Could you check a few things on this model? Use its own coordinates, in mm. Face numbers are marked on the shaded views. Give positions to 0.01 mm unless a question says otherwise; leave off trailing zeros. Order: outer loops, then holes, each group sorted by start corner. A loop starts at its lowest first (then second) coordinate and runs counter-clockwise, first axis right, second up.
(1) If I drill on probe 1 along X at (y, z) = (-11, 14.5); probe 2 along X at (y, z) = (-3, 1.25); probe 3 along Y at (x, z) = (-16, 14.75), over which ranges is the centre line in solid material (lowest first)?
(2) Imagine slicing it at A-A, the plane z = 7. Write out the boundary of the cut face in (x, y) (3 decimals), then the cut area to 3 significant figures.
(3) Imagine slicing it at B-B, the plane z = 1.75. Write out the boundary of the cut face in (x, y) (3 decimals).
(4) Will these pins go through, and if not, where does the flat tip stop? pin 1 (8 mm diameter, centred on x = 8, z = 23, fed in from -Y); pin 2 (3 mm diameter, centred on y = -15, z = 11, fed in from -X); pin 3 (6 mm diameter, centred on x = 1, z = 9.5, fed in from +Y).
(5) If we mould it in two halves opening along X, with no side actions, what happens to the marked faces 1, 2 and 3? For each: released by +X, released by -X, zero draft, split by the parting line, or undercut.
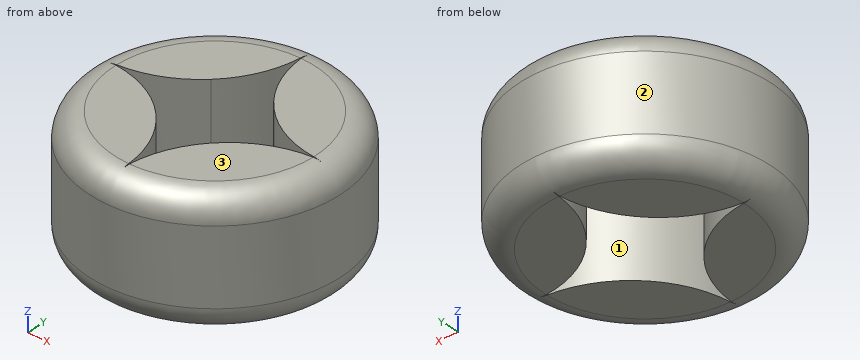
from build123d import *

# Parameters (mm, degrees)
F0_R     = 25.4
F1_DEPTH = 25.4


# Not quite as in the source:
# - a fillet or chamfer that OpenCascade refuses, or shapes differently, is made with other operations: its cross-section is extruded or revolved along the edge and cut away or added


with BuildPart() as f1:
    # F0 (on Top) → F1 (new body)
    with BuildSketch(Plane.XY):
        Circle(F0_R)
        with BuildLine():
            ThreePointArc((0, 22.225), (15.7154482119, 15.7154482119), (22.225, 0))
            ThreePointArc((22.225, 0), (15.7154482119, -15.7154482119), (0, -22.225))
            ThreePointArc((0, -22.225), (-15.7154482119, -15.7154482119), (-22.225, 0))
            ThreePointArc((-22.225, 0), (-15.7154482119, 15.7154482119), (0, 22.225))
        make_face(mode=Mode.SUBTRACT)
        with BuildLine():
            ThreePointArc((-6.5095517729, 6.5095518034), (-1.6917773858, 13.7198607256), (0, 22.225))
            ThreePointArc((0, 22.225), (-15.7154482119, 15.7154482119), (-22.225, 0))
            ThreePointArc((-22.225, 0), (-13.7198607057, 1.6917773941), (-6.5095517729, 6.5095518034))
        make_face()
        with BuildLine():
            ThreePointArc((6.509551813, 6.5095517633), (13.7198607319, 1.6917773832), (22.225, 0))
            ThreePointArc((22.225, 0), (15.7154482119, 15.7154482119), (0, 22.225))
            ThreePointArc((0, 22.225), (1.6917773967, 13.7198606994), (6.509551813, 6.5095517633))
        make_face()
        with BuildLine():
            ThreePointArc((-22.225, 0), (-15.7154482119, -15.7154482119), (0, -22.225))
            ThreePointArc((0, -22.225), (-1.6917773909, -13.7198607133), (-6.5095517917, -6.5095517845))
            ThreePointArc((-6.5095517917, -6.5095517845), (-13.719860718, -1.691777389), (-22.225, 0))
        make_face()
        with BuildLine():
            ThreePointArc((0, -22.225), (15.7154482119, -15.7154482119), (22.225, 0))
            ThreePointArc((22.225, 0), (13.7198607157, -1.6917773899), (6.5095517881, -6.5095517881))
            ThreePointArc((6.5095517881, -6.5095517881), (1.6917773899, -13.7198607157), (0, -22.225))
        make_face()
    extrude(amount=F1_DEPTH)

    # F2: fillet of radius 5.08 on 2 edges, made by hand

    # F2_s1 → F2_t2 (revolve, cut)
    with BuildSketch(Plane.XZ):
        with BuildLine():
            ThreePointArc((25.4, 20.32), (23.9121024484, 23.9121024484), (20.32, 25.4))
            Line((20.32, 25.4), (25.4, 25.4))
            Line((25.4, 25.4), (25.4, 20.32))
        make_face()
    revolve(axis=Axis((0, 0, 25.4), (0, 0, 1)), mode=Mode.SUBTRACT)

    # F2_s3 → F2_t4 (revolve, cut)
    with BuildSketch(Plane.XZ):
        with BuildLine():
            ThreePointArc((25.4, 5.08), (23.9121024484, 1.4878975516), (20.32, 0))
            Line((20.32, 0), (25.4, 0))
            Line((25.4, 0), (25.4, 5.08))
        make_face()
    revolve(axis=Axis((0, 0, 0), (0, 0, 1)), mode=Mode.SUBTRACT)


solid = f1.part
Answer block:
1. probe 1: x = -22.89 to -3.04, 3.04 to 22.89
1. probe 2: x = -23.47 to -11.07, 11.07 to 23.47
1. probe 3: y = -19.73 to -0.89, 0.89 to 19.73
2. outline: circle Ø50.8 at (0, 0); hole (-22.225, 0) arc R22.225 cw to (0, -22.225) arc R22.225 cw to (22.225, 0) arc R22.225 cw to (0, 22.225) arc R22.225 cw to start
2. area: 1,600 mm2
3. outline: circle Ø48.313 at (0, 0); hole (-22.225, 0) arc R22.225 cw to (0, -22.225) arc R22.225 cw to (22.225, 0) arc R22.225 cw to (0, 22.225) arc R22.225 cw to start
4. pin 1: stops at y = -24.95
4. pin 2: stops at x = -21.52
4. pin 3: stops at y = 25.4
5. face 1: undercut
5. face 2: split by the parting line
5. face 3: zero draft
